Model file for the job. Use its own axes, mm. Coordinates: 2 decimals unless noted, no trailing zeros. Loops run counter-clockwise (first coordinate to the right, second up) from the corner with the lowest first, then second, coordinate; pieces in that order, holes last.
from build123d import *

# Parameters (mm, degrees)
BOSS_EXTRUDE1_START                        = -1.5
BOSS_EXTRUDE1_DEPTH                        = 3
PIVOTSHAFTHOLE_CUT_DEPTH                   = 26.816661287
PIVOTSHAFTHOLE_CUT_DEPTH_BACK              = 26.816661287
PIVOTSHAFTHOLE_SKETCH_R                    = 2.51
MOUNTHOLESTOENDBLOCKSEEDFODDER_START       = -1.5
MOUNTHOLESTOENDBLOCKSEEDFODDER_OUTLINE_R   = 2.51
MOUNTHOLESTOENDBLOCKSEEDFODDER_DEPTH       = 3
MOUNTHOLESTOENDBLOCKSEED_SKETCH_R          = 1.575
MOUNTHOLESTOENDBLOCKSEED_CUT_DEPTH         = 26.816661287
MOUNTHOLESTOENDBLOCKSEED_PATTERN_START     = -1.5
MOUNTHOLESTOENDBLOCKSEED_PATTERN_OUTLINE_R = 1.575
MOUNTHOLESTOENDBLOCKSEED_PATTERN_DEPTH     = 3
SPRINGANCHORHOLE_CUT_DEPTH                 = 26.816661287
SPRINGANCHORHOLE_CUT_DEPTH_BACK            = 26.816661287
SPRINGANCHORHOLE_SKETCH_R                  = 1


# Read off the part's stored shape, not the designer's step: mountHolesToEndBlockSeedFodder, mountHolesToEndBlockSeed_pattern
with BuildPart() as part:
    # Sketch1 → Boss-Extrude1 (new body)
    with BuildSketch(Plane(origin=(0, 0, 0), x_dir=(0, 0, -1), z_dir=(1, 0, 0)).offset(BOSS_EXTRUDE1_START)):
        with BuildLine():
            Line((2, 24.5), (7.941302937, -17.662790698))
            ThreePointArc((7.941302937, -17.662790698), (3.119056028, -24.394719129), (-3.834772709, -19.898365989))
            Line((-3.834772709, -19.898365989), (-7, -6.69125))
            Line((-7, -6.69125), (-7, 24.5))
            Line((-7, 24.5), (2, 24.5))
        make_face()
    extrude(amount=BOSS_EXTRUDE1_DEPTH)

    # pivotShaftHole_sketch → pivotShaftHole_cut (cut, two sides: drawn at the far end of the back side and taken through both)
    with BuildSketch(Plane(origin=(0, 0, 0), x_dir=(0, 0, -1), z_dir=(1, 0, 0)).offset(-PIVOTSHAFTHOLE_CUT_DEPTH_BACK)):
        with Locations((2, -18.5)):
            Circle(PIVOTSHAFTHOLE_SKETCH_R)
    extrude(amount=PIVOTSHAFTHOLE_CUT_DEPTH + PIVOTSHAFTHOLE_CUT_DEPTH_BACK, mode=Mode.SUBTRACT)

    # mountHolesToEndBlockSeed_pattern outline → mountHolesToEndBlockSeed_pattern (cut)
    with BuildSketch(Plane.YZ.offset(MOUNTHOLESTOENDBLOCKSEED_PATTERN_START)):
        with Locations((-2.49125, 2.5)):
            Circle(MOUNTHOLESTOENDBLOCKSEED_PATTERN_OUTLINE_R)
        with Locations((20.3, 2.5)):
            Circle(MOUNTHOLESTOENDBLOCKSEED_PATTERN_OUTLINE_R)
    extrude(amount=MOUNTHOLESTOENDBLOCKSEED_PATTERN_DEPTH, mode=Mode.SUBTRACT)

    # springAnchorHole_sketch → springAnchorHole_cut (cut, two sides: drawn at the far end of the back side and taken through both)
    with BuildSketch(Plane(origin=(0, 0, 0), x_dir=(0, 0, -1), z_dir=(1, 0, 0)).offset(-SPRINGANCHORHOLE_CUT_DEPTH_BACK)):
        with Locations((2, -4.5)):
            Circle(SPRINGANCHORHOLE_SKETCH_R)
    extrude(amount=SPRINGANCHORHOLE_CUT_DEPTH + SPRINGANCHORHOLE_CUT_DEPTH_BACK, mode=Mode.SUBTRACT)


with BuildPart() as body_2:
    # mountHolesToEndBlockSeedFodder outline → mountHolesToEndBlockSeedFodder (new body)
    with BuildSketch(Plane.YZ.offset(MOUNTHOLESTOENDBLOCKSEEDFODDER_START)):
        with BuildLine():
            Line((24.5, 7), (-6.69125, 7))
            Line((-6.69125, 7), (-19.898365989, 3.834772709))
            ThreePointArc((-19.898365989, 3.834772709), (-24.394719129, -3.119056028), (-17.662790698, -7.941302937))
            Line((-17.662790698, -7.941302937), (24.5, -2))
            Line((24.5, -2), (24.5, 7))
        make_face()
        with Locations((-18.5, -2)):
            Circle(MOUNTHOLESTOENDBLOCKSEEDFODDER_OUTLINE_R, mode=Mode.SUBTRACT)
    extrude(amount=MOUNTHOLESTOENDBLOCKSEEDFODDER_DEPTH)

    # mountHolesToEndBlockSeed_sketch → mountHolesToEndBlockSeed_cut (cut, symmetric)
    with BuildSketch(Plane(origin=(0, 0, 0), x_dir=(0, 0, -1), z_dir=(1, 0, 0))):
        Circle(MOUNTHOLESTOENDBLOCKSEED_SKETCH_R)
    extrude(amount=MOUNTHOLESTOENDBLOCKSEED_CUT_DEPTH, both=True, mode=Mode.SUBTRACT)


solid = part.part
Q1. Slice it at D-D (y = -4.5). List the corners of the cut face in (x, z).
Answers:
outline: (-1.5, -6.09) - (1.5, -6.09) - (1.5, -3) - (-1.5, -3) - close; (-1.5, -1) - (1.5, -1) - (1.5, 7) - (-1.5, 7) - close
Q2. Slice it at A-A (y = -18.5). List the corners of the cut face in (x, z), and give its area (3 significant figures).
Answers:
outline: (-1.5, -8) - (1.5, -8) - (1.5, -4.51) - (-1.5, -4.51) - close; (-1.5, 0.51) - (1.5, 0.51) - (1.5, 4.17) - (-1.5, 4.17) - close
area: 21.4 mm2
Q3. Drill centre lines: line 1 (Y direction, x = 0.65, z = 3.25); line 2 (Y direction, x = -1.3, z = 1.5); line 3 (Z direction, x = -0.15, y = -2.5). Where is each one in solid material? Low to high.
Answers:
line 1: y = -21.4 to -3.88, -1.11 to 18.92, 21.68 to 24.5
line 2: y = -23.37 to -3.71, -1.27 to 19.08, 21.52 to 24.5
line 3: z = -5.8 to 0.93, 4.07 to 7
Q4. Slice it at C-C (z = 2.5). List the corners of the cut face in (x, y) (3 decimals), and give its area (3 significant figures).
Answers:
outline: (-1.5, -22.469) - (1.5, -22.469) - (1.5, -4.066) - (-1.5, -4.066) - close; (-1.5, -0.916) - (1.5, -0.916) - (1.5, 18.725) - (-1.5, 18.725) - close; (-1.5, 21.875) - (1.5, 21.875) - (1.5, 24.5) - (-1.5, 24.5) - close
area: 122 mm2
Q5. Mould opens along Y. For faces 1 (the flat face through (0, 9, 7)), 2 (the flat face through (-0.02, 3.71, -4.93)), 3 (the flat face through (-0.021, -13.387, 5.395)), 4 (the cylindrical face through (-0.02, -20.95, -1.46)) say: +Y half, -Y half, draft (parallel to the pull), parting line (faces both ways), or undercut.
Answers:
face 1: draft
face 2: +Y half
face 3: -Y half
face 4: undercut
Q6. Slice it at B-B (x = 0.15). List the corners of the cut face in (y, z) (3 decimals), and give its area (3 significant figures).
Answers:
outline: (-19.898, 3.835) arc R6 ccw to (-17.663, -7.941) - (24.5, -2) - (24.5, 7) - (-6.691, 7) - close; hole circle Ø5.02 at (-18.5, -2); hole circle Ø2 at (-4.5, -2); hole circle Ø3.15 at (-2.491, 2.5); hole circle Ø3.15 at (20.3, 2.5)
area: 519 mm2
Q7. Flat gauge pins, fed straight in: P1, Ø1.5, axis at y = 9, z = -6, coming from the -X side; P2, Ø8, axis at y = -18.5, z = -2, coming from the +X side. Where does each tip first touch, or does it go through?
Answers:
P1: passes through
P2: stops at x = 1.5
